Autodesk Fusion 360 part; units mm, degrees
sketch "Schizzo1" plane through (0, 0, 0) normal (0, 0, 1) x (1, 0, 0)
  line L0 (0, 0) -> (-25, 0)
  line L1 (-25, 0) -> (-25, 3)
  line L2 (-25, 3) -> (-5, 3)
  line L3 (-5, 3) -> (-5, 11.5)
  line L4 (-5, 11.5) -> (-25, 11.5)
  line L5 (-25, 11.5) -> (-25, 14.5)
  line L6 (-25, 14.5) -> (0, 14.5)
  line L7 (0, 14.5) -> (0, 0)
  line L8 (0, 14.5) -> (25, 14.5)
  line L9 (5, 11.5) -> (5, 3)
  line L10 (0, 0) -> (0, 14.5)
  line L11 (25, 0) -> (0, 0)
  line L12 (5, 3) -> (25, 3)
  line L13 (25, 14.5) -> (25, 11.5)
  line L14 (25, 3) -> (25, 0)
  line L15 (25, 11.5) -> (5, 11.5)
  line L16 (7.25, 0) -> (7.25, -25)
  line L17 (4.25, -5) -> (-4.25, -5)
  line L18 (4.25, -25) -> (4.25, -5)
  line L19 (-7.25, -25) -> (-7.25, 0)
  line L20 (-4.25, -5) -> (-4.25, -25)
  line L21 (-4.25, -25) -> (-7.25, -25)
  line L22 (7.25, -25) -> (4.25, -25)
  line L23 (0, 0) -> (0, -13.3515) construction
  point P0 (0, 14.5)
  point P1 (0, -5)
  dimension "d2" = 8.5
  dimension "d3" = 3
  dimension "d4" = 3
  dimension "d5" = 25
  dimension "d6" = 25
  dimension "d7" = 20
  dimension "d8" = 8.5
  dimension "d9" = 3
  dimension "d10" = 3
  dimension "d11" = 25
  dimension "d12" = 25
  dimension "d23" = 3
  dimension "d24" = 25
  dimension "d25" = 25
  dimension "d26" = 8.5
  dimension "d27" = 3
  dimension "d28" = 20
  dimension "d31" = 5
  dimension "d34" = 4.25
  dimension "d35" = 20
extrude "Estrusione1" add sketch "Schizzo1" along normal blind 250
fillet "Raccordo2" radius 10 2 edges at (-7.25, 0, 125) (7.25, 0, 125)
equation "d34 = ( 8.5 / 2 ) * 1 mm"
The model under review builds one solid part; all positions refer to its coordinate system, in mm. A direction names the side the tool comes from. Give positions to 0.01 mm unless a question says otherwise; leave off trailing zeros. Loops run counter-clockwise (first coordinate to the right, second up) from the corner with the lowest first, then second, coordinate; pieces in that order, holes last. Notation, with made-up numbers: (48, -10.5) -> (93, -10.5) arc R18 cw to (93, 13.5) -> close; hole circle Ø6 at (88.25, 5.5). An arc over 180 degrees is marked (long way). Put each result on its own line as item: value. Start each with the question number.
1. For faces 1 (the face through (-15, 11.5, 123)), 2 (the face through (-4.25, -15, 123)), 3 (the face through (7.25, -17, 123)), 4 (the face through (-21, 0, 123)), list the 3-axis set-ups (+Z, -Z, +X, -X, +Y, -Y) from which the entire face can be reached by the end or side of a thin tool; tool diameter is ignored.
2. We need section D-D on y = 6. State the section outline as (x, z) points, then the cut area to 3 significant figures.
3. Mouldability with a two-part tool opening along X and no side actions: class faces 5 (the face through (5, 7, 123)), 6 (the face through (4.25, -15, 123)), 7 (the face through (15, 11.5, 123)), 8 (the face through (0, -5, 123)) as released by +X, released by -X, zero draft, split by the parting line, or undercut.
4. We need section B-B on y = -14.5. State the section outline as (x, z) points, then the cut area to 3 significant figures.
5. Clearance check with flat-ended pins moving along their axes: P1, Ø1.5, axis at x = 10.5, z = 149.5, coming from the -Y side; P2, Ø3, axis at y = 9.5, z = 140, coming from the +X side; P3, Ø10, axis at y = -11, z = 162, coming from the -X side. State where each tip first meets the part, or that it passes through.
6. We need section A-A on x = -20.5. State the section outline as (y, z) points.
7. Wall thickness on probe 1 along Y at (x, z) = (-6, 167.5); probe 2 along Y at (x, z) = (19, 20); probe 3 along X at (y, z) = (-12.5, 80.5): over which ranges is each line inside the solid? List them lowest first.
8. We need section C-C on z = 226. State the section outline as (x, y) points.
Determined:
1. face 1: +Z, -Z, -X
1. face 2: +Z, -Z, -Y
1. face 3: +Z, -Z, +X, -Y
1. face 4: +Z, -Z, -X, -Y
2. outline: (-5, 0) -> (5, 0) -> (5, 250) -> (-5, 250) -> close
2. area: 2,500 mm^2
3. face 5: released by +X
3. face 6: undercut
3. face 7: zero draft
3. face 8: undercut
4. outline: (-7.25, 0) -> (-4.25, 0) -> (-4.25, 250) -> (-7.25, 250) -> close; (4.25, 0) -> (7.25, 0) -> (7.25, 250) -> (4.25, 250) -> close
4. area: 1,500 mm^2
5. P1: y = -3.39
5. P2: x = 5
5. P3: x = -8.08
6. outline: (0, 0) -> (3, 0) -> (3, 250) -> (0, 250) -> close; (11.5, 0) -> (14.5, 0) -> (14.5, 250) -> (11.5, 250) -> close
7. probe 1: -25 to 3, 11.5 to 14.5
7. probe 2: 0 to 3, 11.5 to 14.5
7. probe 3: -7.25 to -4.25, 4.25 to 7.25
8. outline: (-25, 0) -> (-17.25, 0) arc R10 cw to (-7.25, -10) -> (-7.25, -25) -> (-4.25, -25) -> (-4.25, -5) -> (4.25, -5) -> (4.25, -25) -> (7.25, -25) -> (7.25, -10) arc R10 cw to (17.25, 0) -> (25, 0) -> (25, 3) -> (5, 3) -> (5, 11.5) -> (25, 11.5) -> (25, 14.5) -> (-25, 14.5) -> (-25, 11.5) -> (-5, 11.5) -> (-5, 3) -> (-25, 3) -> close
